CAD build for the part. Positions are in the model's coordinates, mm. Face numbers are marked on the shaded views. A direction names the side the tool comes from. Give positions to 0.01 mm unless a question says otherwise; leave off trailing zeros. Write each loop counter-clockwise with the first axis right and the second up, starting at its lowest first coordinate (ties: lowest second). Pieces come first, ordered by that corner, then holes. Notation, with made-up numbers: (-4.5, -22) -> (14.5, -22) arc R30 cw to (14.5, 1) -> close; hole circle Ø5 at (-2.5, 44.25). An arc over 180 degrees is marked (long way). Answer in a Markdown table with one row per item. Add a question column.
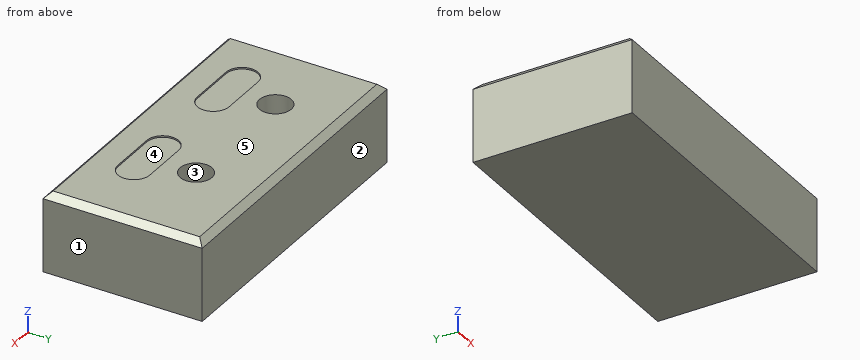
```python
from build123d import *

# Parameters (mm, degrees)
F0_W     = 96.38
F0_H     = 50
F1_DEPTH = 25
F2_R     = 5
F3_DEPTH = 6.5
F4_R     = 1
F5_DEPTH = 22
F6_SIZE  = 2
F8_DEPTH = 0.5


with BuildPart() as f1:
    # F0 (on Top) → F1 (new body)
    with BuildSketch(Plane.XY):
        with Locations((48.19, 25)):
            Rectangle(F0_W, F0_H)
    extrude(amount=F1_DEPTH)

    # F2 (on face) → F3 (cut)
    with BuildSketch(Plane.XY.offset(25)):
        with Locations((25, 30)):
            Circle(F2_R)
        with Locations((66.38, 30)):
            Circle(F2_R)
    extrude(amount=-F3_DEPTH, mode=Mode.SUBTRACT)

    # F4 (on face) → F5 (cut)
    with BuildSketch(Plane.XY.offset(25)):
        with Locations((66.38, 30)):
            Circle(F4_R)
    extrude(amount=-F5_DEPTH, mode=Mode.SUBTRACT)

    # F6
    f6_edges = [f1.edges().sort_by_distance(p)[0] for p in [
        (48.19, 0, 25),
        (96.38, 25, 25),
        (0, 25, 25),
        (48.19, 50, 25),
    ]]
    chamfer(f6_edges, length=F6_SIZE)

    # F7 (on face) → F8 (cut)
    with BuildSketch(Plane.XY.offset(25)):
        with BuildLine():
            Line((32.5, 20), (17.5, 20))
            ThreePointArc((17.5, 20), (13.964466, 18.535534), (12.5, 15))
            ThreePointArc((12.5, 15), (13.964466, 11.464466), (17.5, 10))
            Line((17.5, 10), (32.5, 10))
            ThreePointArc((32.5, 10), (36.035534, 11.464466), (37.5, 15))
            ThreePointArc((37.5, 15), (36.035534, 18.535534), (32.5, 20))
        make_face()
        with BuildLine():
            Line((73.88, 20), (58.88, 20))
            ThreePointArc((58.88, 20), (55.344466, 18.535534), (53.88, 15))
            ThreePointArc((53.88, 15), (55.344466, 11.464466), (58.88, 10))
            Line((58.88, 10), (73.88, 10))
            ThreePointArc((73.88, 10), (77.415534, 11.464466), (78.88, 15))
            ThreePointArc((78.88, 15), (77.415534, 18.535534), (73.88, 20))
        make_face()
    extrude(amount=-F8_DEPTH, mode=Mode.SUBTRACT)


solid = f1.part
```
Item 1: Which spindle directions (+Z, -Z, +X, -X, +Y, -Y) get a long thin tool onto all of the face, cutting with end or side? Do the marked faces 4 and 5. Say none if no direction does.
Item 2: Slice it at A-A, the plane y = 30. List the corners of the cut face in (x, z), then the cut area to 3 significant figures.
Item 3: Slice it at B-B, the plane z = 21. List the corners of the cut face in (x, y), then the cut area to 3 significant figures.
Item 4: Probe L1, parallel to Y at x = 66.38, z = 9.75; L2, parallel to Y at x = 66.38, z = 23; L3, parallel to Z at x = 67, y = 33. List the from-to ranges inside material, lowest first. Write a range as from..to.
Item 5: Drop flat-ended pins along their axis: pin 1 Ø0.6 at (x, z) = (67, 25) entering from +Y; pin 2 Ø3 at (x, y) = (64.5, 30.5) entering from +Z. Give the stop position or say it passes through.
Item 6: Slice it at C-C, the plane x = 25. List the corners of the cut face in (y, z), then the cut area to 3 significant figures.
Item 7: Mould opens along X. For the marked faces 1, 2 and 3 say: released by +X, released by -X, zero draft, split by the parting line, or undercut.
Item 8: Slice it at D-D, the plane x = 66.38. List the corners of the cut face in (y, z).
Answer key:
| question | item | result |
|---|---|---|
| 1 | face 4 | +Z |
| 1 | face 5 | +Z, +X, -X, +Y, -Y |
| 2 | outline | (0, 0) -> (96.38, 0) -> (96.38, 23) -> (94.38, 25) -> (71.38, 25) -> (71.38, 18.5) -> (67.38, 18.5) -> (67.38, 3) -> (65.38, 3) -> (65.38, 18.5) -> (61.38, 18.5) -> (61.38, 25) -> (30, 25) -> (30, 18.5) -> (20, 18.5) -> (20, 25) -> (2, 25) -> (0, 23) -> close |
| 2 | area | 2,240 mm² |
| 3 | outline | (0, 0) -> (96.38, 0) -> (96.38, 50) -> (0, 50) -> close; hole circle Ø10 at (25, 30); hole circle Ø10 at (66.38, 30) |
| 3 | area | 4,660 mm² |
| 4 | L1 | y = 0..29, 31..50 |
| 4 | L2 | y = 0..25, 35..50 |
| 4 | L3 | z = 0..18.5 |
| 5 | pin 1 | stops at y = 48.3 |
| 5 | pin 2 | stops at z = 18.5 |
| 6 | outline | (0, 0) -> (50, 0) -> (50, 23) -> (48, 25) -> (35, 25) -> (35, 18.5) -> (25, 18.5) -> (25, 25) -> (20, 25) -> (20, 24.5) -> (10, 24.5) -> (10, 25) -> (2, 25) -> (0, 23) -> close |
| 6 | area | 1,180 mm² |
| 7 | face 1 | released by +X |
| 7 | face 2 | zero draft |
| 7 | face 3 | undercut |
| 8 | outline | (0, 0) -> (50, 0) -> (50, 23) -> (48, 25) -> (35, 25) -> (35, 18.5) -> (31, 18.5) -> (31, 3) -> (29, 3) -> (29, 18.5) -> (25, 18.5) -> (25, 25) -> (20, 25) -> (20, 24.5) -> (10, 24.5) -> (10, 25) -> (2, 25) -> (0, 23) -> close |
